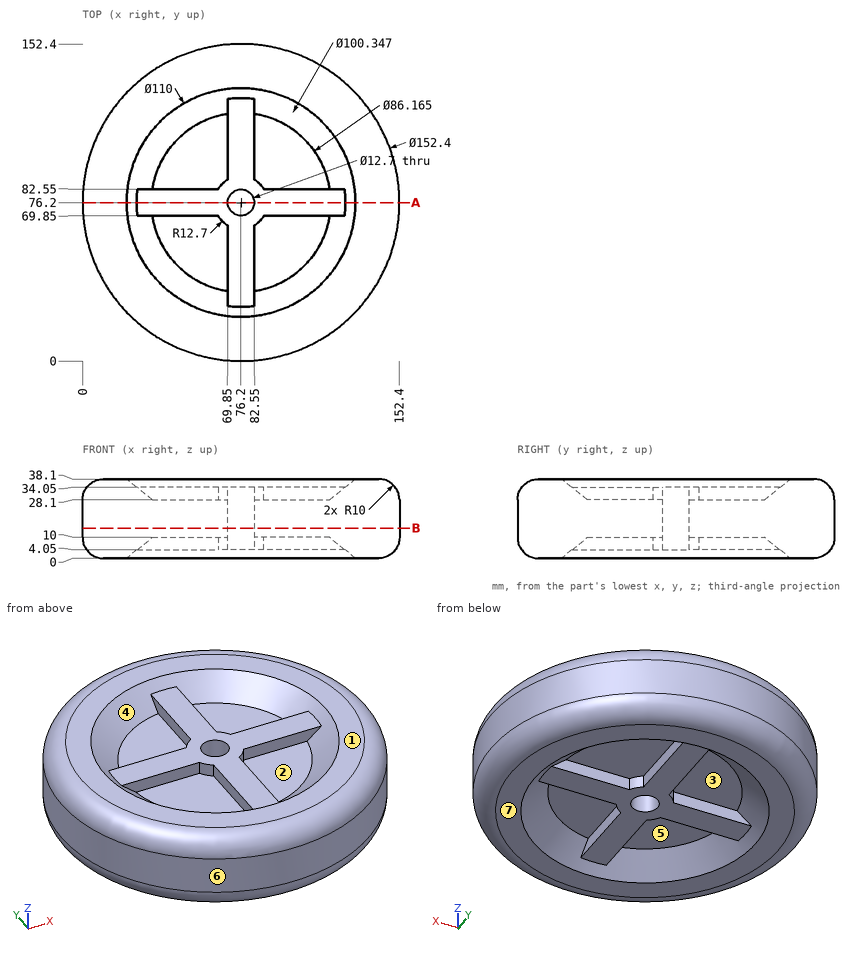
Input: dimensioned drawing with shaded views. Units: mm. Origin: part minimum x, y, z. A direction names the side the tool comes from. Round coordinates to 2 decimals unless told otherwise and drop trailing zeros. Order: outer loops, then holes, each group sorted by start corner. A loop starts at its lowest first (then second) coordinate and runs counter-clockwise, first axis right, second up.
1. Cut plane A-A, the plane y = 76.2. Output: boundary loops of the cut face in (x, z).
The answers:
outline: (0, 10) arc R10 ccw to (10, 0) - (21.2, 0) - (26.03, 4.05) - (69.85, 4.05) - (69.85, 34.05) - (26.03, 34.05) - (21.2, 38.1) - (10, 38.1) arc R10 ccw to (0, 28.1) - close; (82.55, 4.05) - (126.37, 4.05) - (131.2, 0) - (142.4, 0) arc R10 ccw to (152.4, 10) - (152.4, 28.1) arc R10 ccw to (142.4, 38.1) - (131.2, 38.1) - (126.37, 34.05) - (82.55, 34.05) - close
2. Pin query (flat end, axial travel): P1, Ø3, axis at x = 44, z = 31, coming from the -Y side; P2, Ø5, axis at y = 53, z = 7, coming from the -X side; P3, Ø11, axis at x = 46, y = 107.5, coming from the +Z side; P4, Ø3, axis at x = 45.5, y = 19, coming from the -Z side. Return the tip coordinate at first contact, or that it passes through.
The answers:
P1: stops at y = 6.8
P2: stops at x = 3.12
P3: stops at z = 33.06
P4: stops at z = 0
3. Cut plane B-B, the plane z = 14.5. Output: boundary loops of the cut face in (x, y), then the cut area to 3 significant figures.
The answers:
outline: circle Ø152.4 at (76.2, 76.2); hole circle Ø12.7 at (76.2, 76.2)
area: 18,100 mm2
4. Material intervals for line 1 (Y direction, x = 76, z = 20); line 2 (Z direction, x = 102, y = 84.5), sorted ascending.
The answers:
line 1: y = 0 to 69.85, 82.55 to 152.4
line 2: z = 10 to 28.1
5. Set-up query: the marked faces 1, 2 and 3. Return all of +Z, -Z, +X, -X, +Y, -Y with unobstructed straight access to the full face (end or side cutting, diameter ignored); none if empty.
The answers:
face 1: +Z, +X, -X, +Y, -Y
face 2: +Z
face 3: -Z
6. Mould query, pull axis Y, two halves, no side actions, for the marked faces 4, 5, 6 and 7. Classes: released by +Y, released by -Y, zero draft, split by the parting line, or undercut.
The answers:
face 4: undercut
face 5: undercut
face 6: split by the parting line
face 7: zero draft
